The listing builds one solid part. Answer for the finished solid, in the listing's coordinates (mm). A direction names the side the tool comes from. Give positions to 0.01 mm unless a question says otherwise; leave off trailing zeros. Order: outer loops, then holes, each group sorted by start corner. A loop starts at its lowest first (then second) coordinate and runs counter-clockwise, first axis right, second up. Notation, with made-up numbers: (-5, 19) - (36, 19) arc R18 cw to (36, 54) - close; hole circle Ø8 at (84, 83.5). An arc over 180 degrees is marked (long way). Answer in a Markdown table with one row per item.
from build123d import *

# Parameters (mm, degrees)
SKETCH1_R           = 6
BOSS_EXTRUDE1_DEPTH = 17.5
SKETCH2_R           = 6
SKETCH2_R_2         = 5.25
BOSS_EXTRUDE2_DEPTH = 20


with BuildPart() as part:
    # Sketch1 → Boss-Extrude1 (new, symmetric)
    with BuildSketch(Plane.XY):
        Circle(SKETCH1_R)
        with BuildLine():
            Line((1.55, -5.015974482), (1.55, -3.585195962))
            Line((1.55, -3.585195962), (0.55, -3.585195962))
            Line((0.55, -3.585195962), (0.55, -5.221110993))
            Line((0.55, -5.221110993), (-0.55, -5.221110993))
            Line((-0.55, -5.221110993), (-0.55, -3.585195962))
            Line((-0.55, -3.585195962), (-1.55, -3.585195962))
            Line((-1.55, -3.585195962), (-1.55, -5.015974482))
            ThreePointArc((-1.55, -5.015974482), (-5.25, 0), (-1.55, 5.015974482))
            Line((-1.55, 5.015974482), (-1.55, 3.585195962))
            Line((-1.55, 3.585195962), (-0.55, 3.585195962))
            Line((-0.55, 3.585195962), (-0.55, 5.221110993))
            Line((-0.55, 5.221110993), (0.55, 5.221110993))
            Line((0.55, 5.221110993), (0.55, 3.585195962))
            Line((0.55, 3.585195962), (1.55, 3.585195962))
            Line((1.55, 3.585195962), (1.55, 5.015974482))
            ThreePointArc((1.55, 5.015974482), (5.25, 0), (1.55, -5.015974482))
        make_face(mode=Mode.SUBTRACT)
    extrude(amount=BOSS_EXTRUDE1_DEPTH, both=True)

    # Sketch2 → Boss-Extrude2 (add)
    with BuildSketch(Plane(origin=(0, 0, -17.5), x_dir=(-1, 0, 0), z_dir=(0, 0, -1))):
        Circle(SKETCH2_R)
        Circle(SKETCH2_R_2, mode=Mode.SUBTRACT)
    extrude(amount=BOSS_EXTRUDE2_DEPTH)


solid = part.part
Item 1: Each of these flat-tipped pins is pushed along its axis until it touches: P1, Ø1.3, axis at y = -4.5, z = 7.5, coming from the -X side; P2, Ø1.1, axis at x = 1, z = 4, coming from the -Y side; P3, Ø0.5, axis at x = -1, z = -5, coming from the +Y side. Where does it stop, or does it pass through?
Answer block:
| item | result |
|---|---|
| P1 | x = -4.6 |
| P2 | y = -5.98 |
| P3 | y = 5.95 |
Item 2: Find section C-C on z = -8. Write down the section's boundary in (x, y).
Answer block:
| item | result |
|---|---|
| outline | circle Ø12 at (0, 0); hole (-1.55, -5.02) - (-1.55, -3.59) - (-0.55, -3.59) - (-0.55, -5.22) - (0.55, -5.22) - (0.55, -3.59) - (1.55, -3.59) - (1.55, -5.02) arc R5.25 ccw to (1.55, 5.02) - (1.55, 3.59) - (0.55, 3.59) - (0.55, 5.22) - (-0.55, 5.22) - (-0.55, 3.59) - (-1.55, 3.59) - (-1.55, 5.02) arc R5.25 ccw to start |
Item 3: Consider line 1 (X direction, y = 0, z = -10.5); line 2 (X direction, y = 2.25, z = 0.5). Determine where each line is inside the solid, lowest interval first.
Answer block:
| item | result |
|---|---|
| line 1 | -6 to -5.25, 5.25 to 6 |
| line 2 | -5.56 to -4.74, 4.74 to 5.56 |
Item 4: Which of the six approach directions +Z, -Z, +X, -X, +Y, -Y give full straight-line access (tool end or side, diameter ignored) to faces 3 (the face through (-0.55, 4, 0)), 4 (the face through (-4, -4, -37.5)), 5 (the face through (1, -4, -17.5))?
Answer block:
| item | result |
|---|---|
| face 3 | +Z, -Z |
| face 4 | -Z, +X, -X, +Y, -Y |
| face 5 | -Z |
Item 5: Find section A-A on y = 0. Write down the section's boundary in (x, z).
Answer block:
| item | result |
|---|---|
| outline | (-6, -37.5) - (-5.25, -37.5) - (-5.25, 17.5) - (-6, 17.5) - close; (5.25, -37.5) - (6, -37.5) - (6, 17.5) - (5.25, 17.5) - close |
Item 6: Find section D-D on x = -4.75. Write down the section's boundary in (y, z).
Answer block:
| item | result |
|---|---|
| outline | (-3.67, -37.5) - (-2.24, -37.5) - (-2.24, 17.5) - (-3.67, 17.5) - close; (2.24, -37.5) - (3.67, -37.5) - (3.67, 17.5) - (2.24, 17.5) - close |
Item 7: Determine the mould class of faces 1 (the face through (1, 4, 17.5)), 2 (the face through (1, -3.585, 0)) for opening direction Y: pulls with the +Y half, pulls with the -Y half, needs draft (parallel to the pull), parting line crosses it, or undercut.
Answer block:
| item | result |
|---|---|
| face 1 | needs draft |
| face 2 | undercut |
